Study the drawing (mm; zero at the part's minimum x, y, z) and answer. A direction names the side the tool comes from. Coordinates: 2 decimals unless noted, no trailing zeros. Loops run counter-clockwise (first coordinate to the right, second up) from the corner with the lowest first, then second, coordinate; pieces in that order, holes last. Notation, with made-up numbers: (-19, -16) -> (14, -16) arc R21 cw to (14, 19) -> close; hole circle Ø5 at (72, 0). An arc over 180 degrees is marked (long way). One line per question, with ' | ' between items.
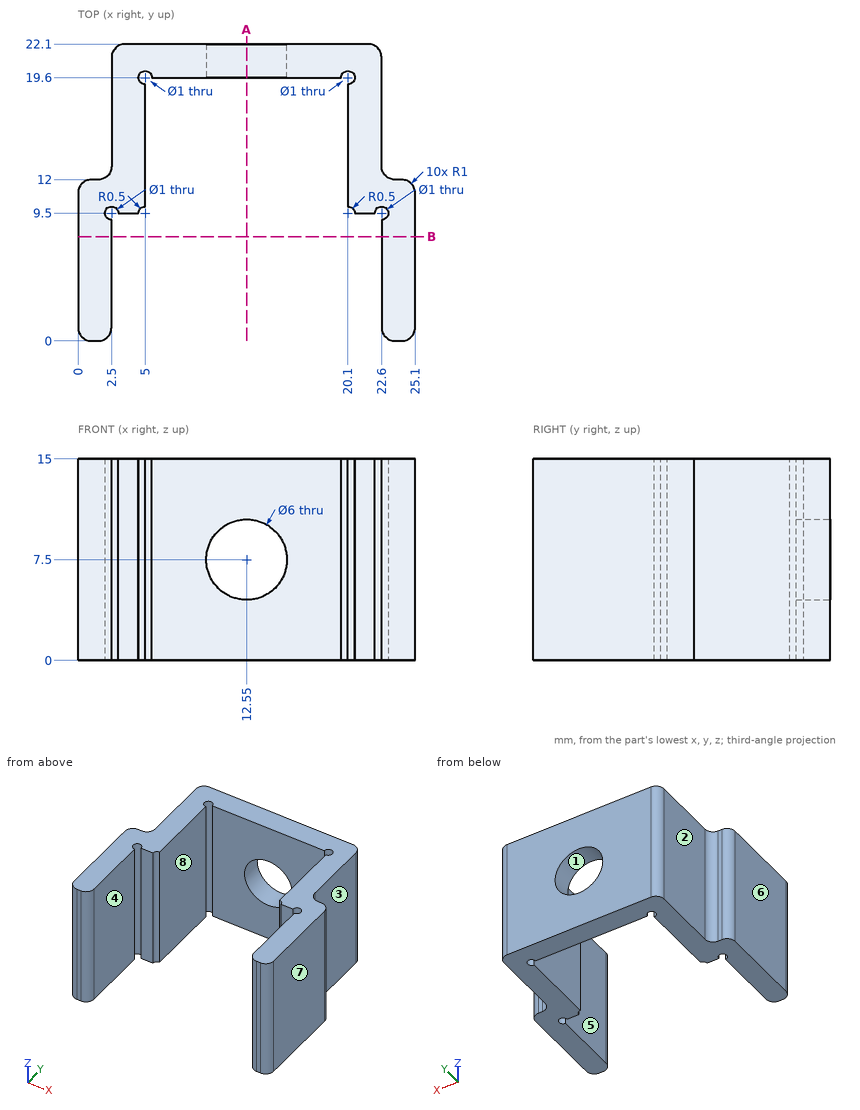
1) Find section B-B (y = 7.75). Write down the section's boundary in (x, z).
Check values:
outline: (0, 0) -> (2.5, 0) -> (2.5, 15) -> (0, 15) -> close; (22.6, 0) -> (25.1, 0) -> (25.1, 15) -> (22.6, 15) -> close
2) Flat-ended cylindrical pins translate along their axes: pin 1 (2 mm diameter, centred on x = 20, z = 4, fed in from -Y); pin 2 (2.5 mm diameter, centred on y = 12.5, z = 7.5, fed in from -X); pin 3 (4 mm diameter, centred on y = 15.5, z = 9.5, fed in from +X). Find the tip coordinate at first contact, or state that the pin passes through.
Check values:
pin 1: stops at y = 9.5 | pin 2: stops at x = 0.03 | pin 3: stops at x = 22.6
3) Find section A-A (x = 12.55). Write down the section's boundary in (y, z).
Check values:
outline: (19.6, 0) -> (22.1, 0) -> (22.1, 4.5) -> (19.6, 4.5) -> close; (19.6, 10.5) -> (22.1, 10.5) -> (22.1, 15) -> (19.6, 15) -> close
4) For the marked faces 1, 2, 3 and 4, determine the directions among +Z, -Z, +X, -X, +Y, -Y from which every point of the face is accessible in a straight line to the end or side of a thin tool.
Check values:
face 1: +Y, -Y | face 2: +Z, -Z, -X, +Y | face 3: +Z, -Z, +X, +Y | face 4: +Z, -Z, -Y
5) Find the intervals of material crossed by line 1 along X through (y, z) = (9.75, 0.5); line 2 along Z through (x, y) = (12.55, 20.3); line 3 along X through (y, z) = (4.25, 10.5), in increasing order.
Check values:
line 1: x = 0 to 2.07, 2.93 to 4.57, 20.53 to 22.17, 23.03 to 25.1 | line 2: z = 0 to 4.5, 10.5 to 15 | line 3: x = 0 to 2.5, 22.6 to 25.1
6) The mould has two halves that part along X. Classify the marked faces 5, 6, 7 and 8: released by +X, released by -X, zero draft, split by the parting line, or undercut.
Check values:
face 5: undercut | face 6: released by -X | face 7: released by +X | face 8: undercut
